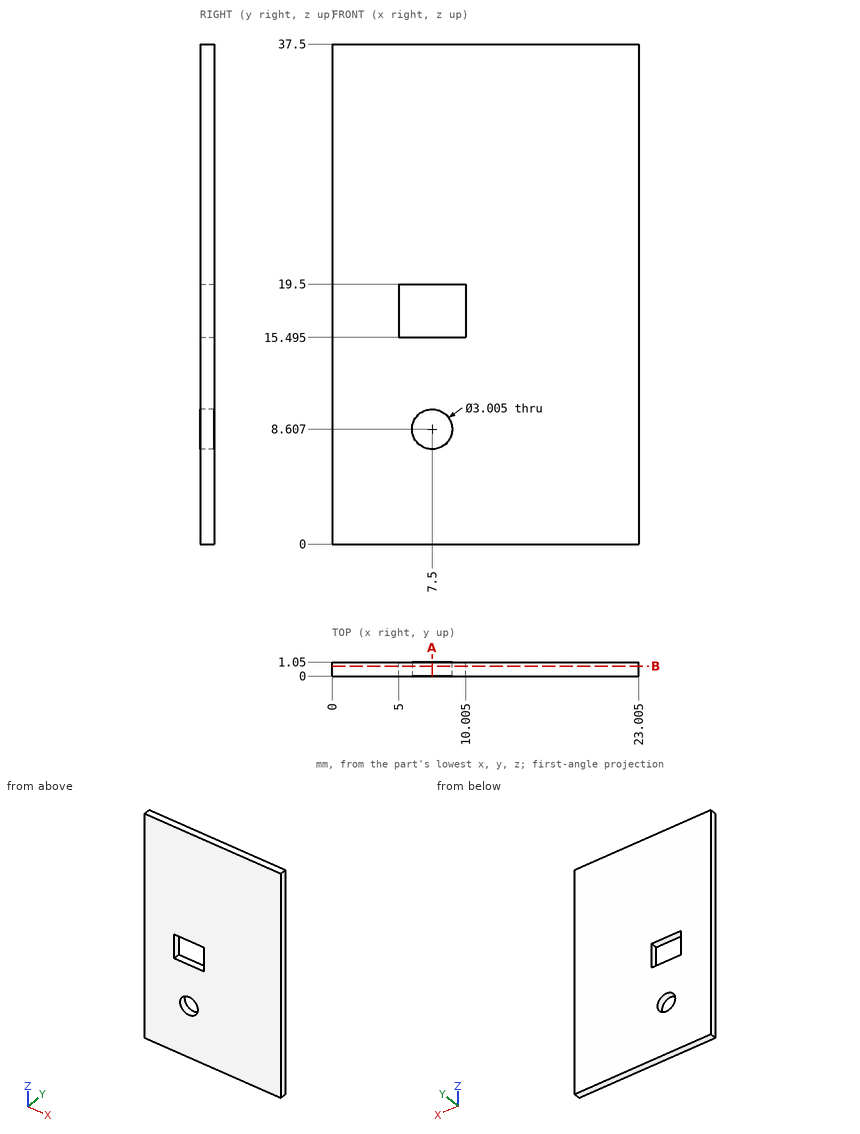
Study the drawing (mm; zero at the part's minimum x, y, z) and answer. Give positions to 0.01 mm unless a question says otherwise; leave off trailing zeros. Write each loop counter-clockwise with the first axis right and the second up, starting at its lowest first coordinate (ties: lowest second). Pieces come first, ordered by that corner, then holes. Notation, with made-up numbers: (59, 1) -> (112, 1) arc R27 ccw to (112, 36) -> close; hole circle Ø9 at (79.25, 69). An arc over 180 degrees is marked (long way). Write item = value, one per line. Start each with the question number.
1) This flat-tipped pin is pushed along its axis until it touches: pin 1 (4 mm diameter, centred on x = 7.5, z = 8.61, fed in from +Y). Where does it stop, or does it pass through?
2) The part is cut by section A-A, the plane x = 7.5. Count the separate pieces of the cut face and the enclosed holes in it, and give its area (3 significant figures).
3) Straight lines are drawn through the part: line 1 along Z through (x, y) = (7.5, 0.4) (1 decimal); line 2 along Z through (x, y) = (7, 0.65) (1 decimal); line 3 along X through (y, z) = (0.15, 17) (1 decimal). For each, find the intervals that lie inside material, in ascending order.
4) The part is cut by section B-B, the plane y = 0.75. Determine the outline of the cut face in (x, z) (1 decimal).
Solutions:
q1.pin_1 = 1.05
q2.separate_pieces = 3
q2.enclosed_holes = 0
q2.area = 32.0 mm²
q3.line_1 = 0 to 7.1, 10.1 to 15.5, 19.5 to 37.5
q3.line_2 = 0 to 7.2, 10 to 15.5, 19.5 to 37.5
q3.line_3 = 0 to 5, 10 to 23
q4.outline = (0, 0) -> (23, 0) -> (23, 37.5) -> (0, 37.5) -> close; hole (5, 15.5) -> (10, 15.5) -> (10, 19.5) -> (5, 19.5) -> close; hole circle Ø3 at (7.5, 8.6)
